```python
from build123d import *

# Parameters (mm, degrees)
ESQUISSE1_W                = 230
ESQUISSE1_H                = 40
BOSS_EXTRU_1_DEPTH         = 5
ESQUISSE2_R                = 2.75
ENL_V_MAT_EXTRU_1_DEPTH    = 117.833214455
ESQUISSE8_R                = 2.75
ENL_V_MAT_EXTRU_2_DEPTH    = 5
R_P_TITION_LIN_AIRE2_COUNT = 5
R_P_TITION_LIN_AIRE2_PITCH = 20
R_P_TITION_LIN_AIRE3_COUNT = 5
R_P_TITION_LIN_AIRE3_PITCH = 20


with BuildPart() as part:
    # Esquisse1 → Boss.-Extru.1 (new body)
    with BuildSketch(Plane.XY):
        Rectangle(ESQUISSE1_W, ESQUISSE1_H)
    extrude(amount=BOSS_EXTRU_1_DEPTH)

    # Esquisse2 → Enlèv. mat.-Extru.1 (cut, through all)
    with BuildSketch(Plane.XY.offset(5)):
        with Locations((20.5, 0)):
            Circle(ESQUISSE2_R)
    enl_v_mat_extru_1 = extrude(amount=-ENL_V_MAT_EXTRU_1_DEPTH, mode=Mode.SUBTRACT)

    # Esquisse8 → Enlèv. mat.-Extru.2 (cut)
    with BuildSketch(Plane(origin=(0, 0, 0), x_dir=(-1, 0, 0), z_dir=(0, 0, -1))):
        with Locations((20.5, 0)):
            Circle(ESQUISSE8_R)
    enl_v_mat_extru_2 = extrude(amount=-ENL_V_MAT_EXTRU_2_DEPTH, mode=Mode.SUBTRACT)

    # Répétition linéaire2: Enlèv. mat.-Extru.1 ×5
    with Locations(*[(i * R_P_TITION_LIN_AIRE2_PITCH, 0, 0) for i in range(1, R_P_TITION_LIN_AIRE2_COUNT)]):
        add(enl_v_mat_extru_1, mode=Mode.SUBTRACT)

    # Répétition linéaire3: Enlèv. mat.-Extru.2 ×5
    with Locations(*[(-i * R_P_TITION_LIN_AIRE3_PITCH, 0, 0) for i in range(1, R_P_TITION_LIN_AIRE3_COUNT)]):
        add(enl_v_mat_extru_2, mode=Mode.SUBTRACT)


solid = part.part
```
Input: part model. Units: mm. Frame: model coordinates. Give positions to 0.01 mm unless a question says otherwise; leave off trailing zeros. Order: outer loops, then holes, each group sorted by start corner. A loop starts at its lowest first (then second) coordinate and runs counter-clockwise, first axis right, second up. Notation, with made-up numbers: (2.25, 38.25) -> (24.25, 38.25) arc R21 cw to (24.25, 49.25) -> close; hole circle Ø3 at (-17, 42). An arc over 180 degrees is marked (long way). Write each question's results on one line, items separated by ' | '. Start each with the question number.
Item 1: Cut plane A-A on x = -40.5. Return the cut outline in (y, z).
Item 2: Line query: line 1 (Y direction, x = -80.5, z = 3.6); line 2 (Y direction, x = -39.5, z = 4.35). Output: solid intervals per line, ascending.
Item 3: Mould query, pull axis Y, two halves, no side actions, for faces 1 (the flat face through (-2, 20, 2)), 2 (the flat face through (-2, 0, 5)), 3 (the cylindrical face through (17.753, 0.121, 2.535)). Classes: pulls with the +Y half, pulls with the -Y half, needs draft (parallel to the pull), parting line crosses it, or undercut.
Item 4: Cut plane B-B on z = 3.9. Give the number of separate pieces and of enclosed holes in the cut face, then the cut area to 3 significant figures.
Item 5: Contact query for flat-ended pins moving along their axis: P1, Ø6.5, axis at x = -40.5, y = 0, coming from the -Z side; P2, Ø4.5, axis at x = 60.5, y = 0, coming from the -Z side. Output: stop coordinate, or through.
Established:
1) outline: (-20, 0) -> (-2.75, 0) -> (-2.75, 5) -> (-20, 5) -> close; (2.75, 0) -> (20, 0) -> (20, 5) -> (2.75, 5) -> close
2) line 1: -20 to -2.75, 2.75 to 20 | line 2: -20 to -2.56, 2.56 to 20
3) face 1: pulls with the +Y half | face 2: needs draft | face 3: undercut
4) separate pieces: 1 | enclosed holes: 10 | area: 8,960 mm^2
5) P1: z = 0 | P2: through
